Can you work these out from the model? Positions are in its coordinate system, mm. A direction names the side the tool comes from. Give positions to 0.01 mm unless a question says otherwise; leave off trailing zeros. Loops run counter-clockwise (first coordinate to the right, second up) from the corner with the lowest first, then second, coordinate; pieces in that order, holes last. Notation, with made-up numbers: (55, -14.5) - (79, -14.5) arc R9 ccw to (79, -0.5) - close; hole circle Ø4 at (61.5, -3.75). An arc over 180 degrees is marked (long way). Answer in a Markdown table with one row per item.
Autodesk Inventor part; units mm, degrees
ref_plane "YZ Plane" through (0, 0, 0) normal (1, 0, 0) x (0, 1, 0)
ref_plane "XZ Plane" through (0, 0, 0) normal (0, 1, 0) x (-1, 0, 0)
ref_plane "XY Plane" through (0, 0, 0) normal (0, 0, 1) x (1, 0, 0)
sketch "Sketch1" plane through (0, 0, 0) normal (1, 0, 0) x (0, 1, 0)
  line L0 (63, -58.6109) -> (63.0005, -43.5826)
  line L1 (60.0005, -43.5825) -> (63.0005, -43.5826)
  line L2 (60.0011, -26.0825) -> (60.0005, -43.5825)
  line L3 (63.0011, -26.0826) -> (60.0011, -26.0825)
  line L4 (63.0011, -26.0826) -> (63.0018, -7.1898)
  line L5 (63.0018, -7.1898) -> (63.0023, 9.6674)
  line L6 (60, 9.6674) -> (63.0023, 9.6674)
  line L7 (60, 27.1674) -> (60, 9.6674)
  line L8 (63, 27.1674) -> (60, 27.1674)
  line L9 (63, 27.1674) -> (63, 44.0245)
  line L10 (63, 44.0245) -> (63, 62.6674)
  line L11 (60, 62.6674) -> (63, 62.6674)
  line L12 (60, 80.1674) -> (60, 62.6674)
  line L13 (63, 80.1674) -> (60, 80.1674)
  line L14 (63, 80.1674) -> (63, 95.2386)
  circle A0 centre (18.25, 69.1244) radius 3.75
  line L15 (16.75, 76.1244) -> (16.75, 75.1244)
  line L16 (17.25, 74.6244) -> (19.25, 74.6244)
  arc A1 (19.25, 74.6244) -> (19.75, 75.1244) centre (19.25, 75.1244) ccw
  line L17 (19.75, 75.1244) -> (19.75, 76.1244)
  arc A2 (19.75, 76.1244) -> (19.25, 76.6244) centre (19.25, 76.1244) ccw
  line L18 (19.25, 76.6244) -> (17.25, 76.6244)
  arc A3 (17.25, 76.6244) -> (16.75, 76.1244) centre (17.25, 76.1244) ccw
  arc A4 (16.75, 75.1244) -> (17.25, 74.6244) centre (17.25, 75.1244) ccw
  circle A5 centre (55.3, -15.9142) radius 1.5875
  circle A6 centre (54.4, -35.289) radius 2.95
  circle A7 centre (47.5, -23.5892) radius 8.25
  circle A8 centre (47.5, -46.9892) radius 8.25
  circle A9 centre (39.7, -54.6642) radius 1.5875
  circle A10 centre (40.6, -35.289) radius 2.95
  circle A11 centre (40.0677, -15.9142) radius 1.5875
  circle A12 centre (55.6677, -54.6642) radius 1.5875
  line L19 (55.3, -15.9142) -> (39.7, -54.6642) construction
  line L20 (55.6677, -54.6642) -> (40.0677, -15.9142) construction
  circle A13 centre (16.9008, -13.4535) radius 9.2
  circle A14 centre (55.3, 90.5858) radius 1.5875
  circle A15 centre (40.0677, 90.5858) radius 1.5875
  circle A16 centre (47.5, 82.9108) radius 8.25
  circle A17 centre (54.4, 71.211) radius 2.95
  circle A18 centre (40.6, 71.211) radius 2.95
  circle A19 centre (47.5, 59.5108) radius 8.25
  circle A20 centre (39.7, 51.8358) radius 1.5875
  circle A21 centre (55.6677, 51.8358) radius 1.5875
  line L21 (55.3, 90.5858) -> (39.7, 51.8358) construction
  line L22 (55.6677, 51.8358) -> (40.0677, 90.5858) construction
  line L23 (3, 8.4171) -> (0, 8.4171)
  line L24 (0, 8.4171) -> (0, 28.4171)
  line L25 (0, 28.4171) -> (3, 28.4171)
  line L26 (3, 28.4171) -> (3, 8.4171) construction
  line L27 (3, 8.4171) -> (0, 28.4171) construction
  line L28 (0, 8.4171) -> (3, 28.4171) construction
  line L29 (31.5, 18.3138) -> (31.5, 31.364) construction
  line L30 (31.5, 18.3138) -> (40.6, 18.3138) construction
  line L31 (3, -21.5829) -> (0, -21.5829)
  line L32 (0, -21.5829) -> (0, -1.5829)
  line L33 (0, -1.5829) -> (3, -1.5829)
  line L34 (3, -51.5829) -> (0, -51.5829)
  line L35 (0, -51.5829) -> (0, -31.5829)
  line L36 (0, -31.5829) -> (3, -31.5829)
  line L37 (3, 38.4171) -> (0, 38.4171)
  line L38 (0, 38.4171) -> (0, 58.4171)
  line L39 (0, 58.4171) -> (3, 58.4171)
  line L40 (3, 8.4171) -> (0, 8.4171)
  line L41 (0, 8.4171) -> (0, 28.4171)
  line L42 (0, 28.4171) -> (3, 28.4171)
  line L43 (3, -21.5829) -> (0, -21.5829)
  line L44 (0, -21.5829) -> (0, -1.5829)
  line L45 (0, -1.5829) -> (3, -1.5829)
  line L46 (3, 68.4171) -> (0, 68.4171)
  line L47 (0, 68.4171) -> (0, 88.4171)
  line L48 (0, 88.4171) -> (3, 88.4171)
  line L49 (3, 38.4171) -> (0, 38.4171)
  line L50 (0, 38.4171) -> (0, 58.4171)
  line L51 (0, 58.4171) -> (3, 58.4171)
  line L52 (3, 8.4171) -> (0, 8.4171)
  line L53 (0, 8.4171) -> (0, 28.4171)
  line L54 (0, 28.4171) -> (3, 28.4171)
  line L55 (3, -51.5829) -> (3, -58.6109)
  line L56 (3, -31.5829) -> (3, -21.5829)
  line L57 (3, -1.5829) -> (3, 8.4171)
  line L58 (3, 28.4171) -> (3, 38.4171)
  line L59 (3, 58.4171) -> (3, 68.4171)
  line L60 (3, 88.4171) -> (3, 95.2386)
  line L61 (28, -58.6109) -> (28, -61.6109)
  line L62 (28, -61.6109) -> (38, -61.6109)
  line L63 (38, -61.6109) -> (38, -58.6109)
  line L64 (38, -58.6109) -> (28, -61.6109) construction
  line L65 (28, -58.6109) -> (38, -61.6109) construction
  line L66 (48, -58.6109) -> (48, -61.6109)
  line L67 (48, -61.6109) -> (58, -61.6109)
  line L68 (58, -61.6109) -> (58, -58.6109)
  line L69 (58, -58.6109) -> (48, -61.6109) construction
  line L70 (48, -58.6109) -> (58, -61.6109) construction
  line L71 (8, -58.6109) -> (8, -61.6109)
  line L72 (8, -61.6109) -> (18, -61.6109)
  line L73 (18, -61.6109) -> (18, -58.6109)
  line L74 (18, -58.6109) -> (8, -61.6109) construction
  line L75 (8, -58.6109) -> (18, -61.6109) construction
  line L76 (28, -58.6109) -> (28, -61.6109)
  line L77 (28, -61.6109) -> (38, -61.6109)
  line L78 (38, -61.6109) -> (38, -58.6109)
  line L79 (38, -58.6109) -> (28, -61.6109) construction
  line L80 (28, -58.6109) -> (38, -61.6109) construction
  line L81 (63, -58.6109) -> (58, -58.6109)
  line L82 (48, -58.6109) -> (38, -58.6109)
  line L83 (28, -58.6109) -> (18, -58.6109)
  line L84 (8, -58.6109) -> (3, -58.6109)
  line L85 (28, 95.2386) -> (28, 98.2386)
  line L86 (28, 98.2386) -> (38, 98.2386)
  line L87 (38, 98.2386) -> (38, 95.2386)
  line L88 (38, 95.2386) -> (28, 98.2386) construction
  line L89 (28, 95.2386) -> (38, 98.2386) construction
  line L90 (58, 98.2386) -> (58, 95.2386)
  line L91 (48, 98.2386) -> (58, 98.2386)
  line L92 (58, 95.2386) -> (48, 98.2386) construction
  line L93 (48, 95.2386) -> (58, 98.2386) construction
  line L94 (48, 95.2386) -> (48, 98.2386)
  line L95 (18, 98.2386) -> (18, 95.2386)
  line L96 (8, 98.2386) -> (18, 98.2386)
  line L97 (18, 95.2386) -> (8, 98.2386) construction
  line L98 (8, 95.2386) -> (18, 98.2386) construction
  line L99 (8, 95.2386) -> (8, 98.2386)
  line L100 (38, 98.2386) -> (38, 95.2386)
  line L101 (28, 98.2386) -> (38, 98.2386)
  line L102 (38, 95.2386) -> (28, 98.2386) construction
  line L103 (28, 95.2386) -> (38, 98.2386) construction
  line L104 (28, 95.2386) -> (28, 98.2386)
  line L105 (48, 95.2386) -> (38, 95.2386)
  line L106 (28, 95.2386) -> (18, 95.2386)
  line L107 (58, 95.2386) -> (63, 95.2386)
  line L108 (8, 95.2386) -> (3, 95.2386)
  point P0 (0, 0)
  point P1 (47.6838, -34.8326)
  point P2 (47.6838, -34.8326)
  point P3 (47.6838, -34.8326)
  point P4 (47.6838, 71.6674)
  point P5 (47.6838, 71.6674)
  point P6 (47.6838, 71.6674)
  point P7 (47.6838, 71.6674)
  point P8 (1.5, 18.4171)
  point P9 (60, 18.4174)
  point P10 (33, -60.1109)
  point P11 (53, -60.1109)
  point P12 (13, -60.1109)
  point P13 (33, -60.1109)
  point P14 (33, 96.7386)
  point P15 (53, 96.7386)
  point P16 (13, 96.7386)
  point P17 (33, 96.7386)
  dimension "d0" = 7.8
  dimension "d1" = 7.8
  dimension "d2" = 7.8
  dimension "d3" = 7.8
  dimension "d7" = 3
  dimension "d8" = 20
  dimension "d11" = 30
  dimension "d14" = 30
  dimension "d17" = 10
  dimension "d18" = 3
  dimension "d21" = 20
  dimension "d24" = 20
extrude "Extrusion1" add sketch "Sketch1" along normal blind 3
properties part number "srf kiri"
Q1. Imagine slicing it at C-C, the plane z = 32. Write out the boundary of the cut face in (x, y).
Checked values:
| item | result |
|---|---|
| outline | (0, 3) - (3, 3) - (3, 63) - (0, 63) - close |
Q2. On a 3-axis mill with a long thin cutter (end or side, diameter ignored), from which of +Z, -Z, +X, -X, +Y, -Y can I reach the whole of each face in a straight line? I mean faces 5 (the face through (1, 38, -60)), 6 (the face through (1, 43, 95.239)), 7 (the face through (1, 1, 28.417)), 8 (the face through (1, 60, 95.239)), 9 (the face through (1, 0, -12)). Say none if no direction works.
Checked values:
| item | result |
|---|---|
| face 5 | -Z, +X, -X |
| face 6 | +Z, +X, -X |
| face 7 | +X, -X, -Y |
| face 8 | +Z, +X, -X, +Y |
| face 9 | +Z, -Z, +X, -X, -Y |
Q3. For pin 1 (8 mm diameter, centred on y = 38.5, z = -34, fed in from -X); pin 2 (0.9 mm diameter, centred on x = 1, z = 85.5, fed in from +Y); pin 3 (0.9 mm diameter, centred on x = 1, y = 62, fed in from +Z); pin 4 (0.9 mm diameter, centred on x = 1, z = 74.5, fed in from +Y), each with a flat end and sliding along its axis, tell me the tip position at first contact or that it passes through.
Checked values:
| item | result |
|---|---|
| pin 1 | stops at x = 0 |
| pin 2 | stops at y = 63 |
| pin 3 | stops at z = 95.24 |
| pin 4 | stops at y = 60 |
Q4. Imagine slicing it at D-D, the plane z = 57. Write out the boundary of the cut face in (x, y), and give its area (3 significant figures).
Checked values:
| item | result |
|---|---|
| outline | (0, 0) - (3, 0) - (3, 39.64) - (0, 39.64) - close; (0, 55.36) - (3, 55.36) - (3, 63) - (0, 63) - close |
| area | 142 mm² |
Q5. Imagine slicing it at A-A, the plane z = -12. Write out the boundary of the cut face in (x, y).
Checked values:
| item | result |
|---|---|
| outline | (0, 0) - (3, 0) - (3, 7.82) - (0, 7.82) - close; (0, 25.99) - (3, 25.99) - (3, 63) - (0, 63) - close |
Q6. If we mould it in two halves opening along Z, with no side actions, what happens to faces 1 (the face through (1, 13, 98.239)), 2 (the face through (1, 63, 45)), 3 (the face through (1, 53, -61.611)), 4 (the face through (1.479, 52.226, -37.283))? For each: released by +Z, released by -Z, zero draft, split by the parting line, or undercut.
Checked values:
| item | result |
|---|---|
| face 1 | released by +Z |
| face 2 | zero draft |
| face 3 | released by -Z |
| face 4 | undercut |
Q7. Imagine slicing it at B-B, the plane y = 45.5. Write out the boundary of the cut face in (x, z), and give its area (3 significant figures).
Checked values:
| item | result |
|---|---|
| outline | (0, -58.61) - (3, -58.61) - (3, -54.99) - (0, -54.99) - close; (0, -38.99) - (3, -38.99) - (3, -31.59) - (0, -31.59) - close; (0, -15.59) - (3, -15.59) - (3, 51.51) - (0, 51.51) - close; (0, 67.51) - (3, 67.51) - (3, 74.91) - (0, 74.91) - close; (0, 90.91) - (3, 90.91) - (3, 95.24) - (0, 95.24) - close |
| area | 269 mm² |
Q8. If I drill on line 1 (Z direction, x = 2.4, y = 47.5); line 2 (Z direction, x = 1.7, y = 44); line 3 (Y direction, x = 2.85, z = 89.5), over which ranges is the centre line in solid material (lowest first)? Write a range as [from, to].
Checked values:
| item | result |
|---|---|
| line 1 | z = [-58.61, -55.24], [-38.74, -31.84], [-15.34, 51.26], [67.76, 74.66], [91.16, 95.24] |
| line 2 | z = [-58.61, -54.46], [-39.52, -31.06], [-16.12, 52.04], [66.98, 75.44], [90.38, 95.24] |
| line 3 | y = [3, 38.91], [41.23, 42.54], [52.46, 54.14], [56.46, 63] |
